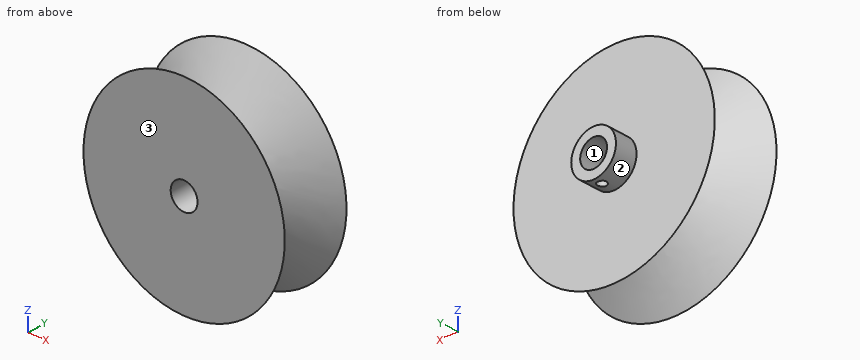
```python
from build123d import *

# Parameters (mm, degrees)
SKETCH3_R               = 5
BOSS_EXTRUDE1_DEPTH     = 5
SKETCH4_R               = 3
CUT_EXTRUDE3_DEPTH      = 20
CUT_EXTRUDE2_REACH      = 39.666
CUT_EXTRUDE2_END_RADIUS = 3
SKETCH6_R               = 1


with BuildPart() as part:
    # Loft1: read off the stored shape, not the designer's step
    # Loft1: loft between two sections, ruled curve by curve
    loft1_from = [
        Edge.make_bspline([(9.916670011, 0, 2.592712073), (15.102094157, 0, -17.240627949), (-4.731245866, 0, -22.426052095), (-9.916670011, 0, -2.592712073), (-15.102094157, 0, 17.240627949), (4.731245866, 0, 22.426052095), (9.916670011, 0, 2.592712073)], [0, 0, 0, 0, 0.5, 0.5, 0.5, 1, 1, 1, 1], 3, [1, 0.333333333, 0.333333333, 1, 0.333333333, 0.333333333, 1]),
    ]
    loft1_to = [
        Edge.make_bspline([(22.487991734, 7.5, 0.735001896), (23.957995526, 7.5, -44.240981571), (-21.017987942, 7.5, -45.710985363), (-22.487991734, 7.5, -0.735001896), (-23.957995526, 7.5, 44.240981571), (21.017987942, 7.5, 45.710985363), (22.487991734, 7.5, 0.735001896)], [0, 0, 0, 0, 0.5, 0.5, 0.5, 1, 1, 1, 1], 3, [1, 0.333333333, 0.333333333, 1, 0.333333333, 0.333333333, 1]),
    ]
    loft1 = Solid(Shell([*[Face.make_surface_from_curves(loft1_from[k], loft1_to[k]) for k in range(1)], Face(Wire(loft1_from)), Face(Wire(loft1_to))]))
    add(loft1)

    # Mirror1: Loft1 across plane
    add(loft1.mirror(Plane.ZX))

    # Sketch3 → Boss-Extrude1 (add)
    with BuildSketch(Plane(origin=(0, 7.5, 0), x_dir=(1, 0, 0), z_dir=(0, 1, 0))):
        with Locations(Location((0, 0, 0), (0, 0, 270))):
            Circle(SKETCH3_R)
    extrude(amount=BOSS_EXTRUDE1_DEPTH)

    # Sketch4 → Cut-Extrude3 (cut)
    with BuildSketch(Plane(origin=(0, 12.5, 0), x_dir=(1, 0, 0), z_dir=(0, 1, 0))):
        with Locations(Location((0, 0, 0), (0, 0, 270))):
            Circle(SKETCH4_R)
    extrude(amount=-CUT_EXTRUDE3_DEPTH, mode=Mode.SUBTRACT)

    # Cut-Extrude2: up to this cylinder (the profile starts outside it)
    cut_extrude2_end = Plane(origin=(0, 10.5, 0), z_dir=(0, 1, 0)) * Cylinder(CUT_EXTRUDE2_END_RADIUS, 86.332, mode=Mode.PRIVATE)
    # Sketch6 → Cut-Extrude2 (cut, up to the surface)
    with BuildSketch(Plane.XY.offset(-5), mode=Mode.PRIVATE) as cut_extrude2_sk1:
        with Locations(Location((0, 10.5, 0), (0, 0, 180))):
            Circle(SKETCH6_R)
    cut_extrude2_tool1 = extrude(cut_extrude2_sk1.sketch, amount=CUT_EXTRUDE2_REACH, mode=Mode.PRIVATE) - cut_extrude2_end
    add(cut_extrude2_tool1.solids().sort_by_distance((0, 10.5, -5))[0], mode=Mode.SUBTRACT)


solid = part.part
```
Source: CAD feature listing. Evaluate the final solid. Frame: model axes, mm. Face numbers are marked on the shaded views. Round coordinates to 2 decimals unless told otherwise and drop trailing zeros. Loops run counter-clockwise (first coordinate to the right, second up) from the corner with the lowest first, then second, coordinate; pieces in that order, holes last.
1. Mould query, pull axis X, two halves, no side actions, for the marked faces 1, 2 and 3. Classes: released by +X, released by -X, zero draft, split by the parting line, or undercut.
2. Contact query for flat-ended pins moving along their axis: pin 1 (12 mm diameter, centred on x = -3.5, z = -13, fed in from +Y); pin 2 (6 mm diameter, centred on y = 1.5, z = 5, fed in from +X); pin 3 (2.5 mm diameter, centred on x = 0, y = 10.5, fed in from -Z). Output: stop coordinate, or through.
3. Ray query, L1, parallel to Y at x = 21, z = -7; L2, parallel to Z at x = 4, y = 9.25; L3, parallel to X at y = 4, z = 0. Return the intervals inside material, ascending.
4. Section query A-A on x = 0. Give the number of separate pieces and of enclosed holes in the cut face, and give its area (3 significant figures).
5. Section query B-B on y = 10.5. Output: boundary loops of the cut face in (x, z), and give its area (3 significant figures).
Answers below:
1. face 1: undercut
1. face 2: split by the parting line
1. face 3: zero draft
2. pin 1: stops at y = 7.5
2. pin 2: stops at x = 16.86
2. pin 3: stops at z = -5
3. L1: y = -7.5 to -7.28, 7.28 to 7.5
3. L2: z = -3 to 3
3. L3: x = -16.7 to -3, 3 to 16.7
4. separate pieces: 3
4. enclosed holes: 0
4. area: 415 mm2
5. outline: (-1, -4.9) - (-1, -2.83) arc R3 cw (long way) to (1, -2.83) - (1, -4.9) arc R5 ccw (long way) to start
5. area: 46.2 mm2
